Drawing for the job (mm, zero at the part's lowest x, y, z). A direction names the side the tool comes from. Coordinates: 2 decimals unless noted, no trailing zeros. Loops run counter-clockwise (first coordinate to the right, second up) from the corner with the lowest first, then second, coordinate; pieces in that order, holes last. Notation, with made-up numbers: (20.5, 40) - (59.5, 40) arc R18 cw to (59.5, 71) - close; hole circle Ø6 at (-13, -13.5). An arc over 180 degrees is marked (long way). Put each result on its own line as item: value.
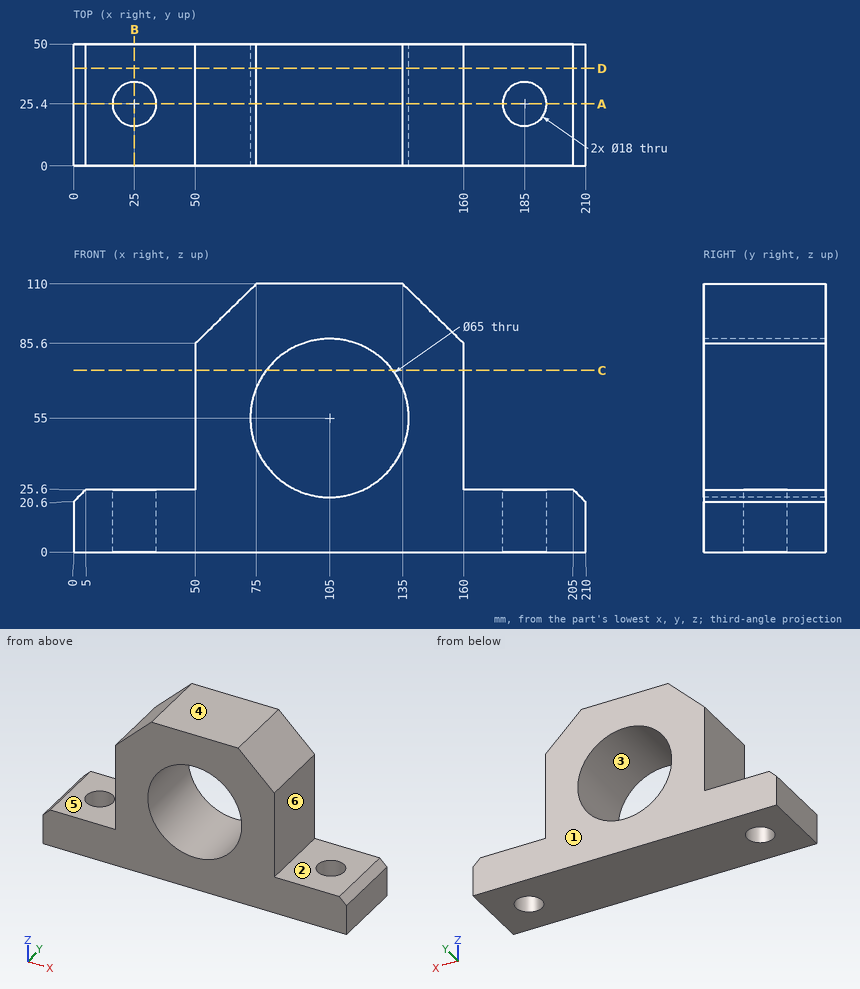
Q1. Tool access for the marked faces 4, 5 and 6: list every direction of +Z, -Z, +X, -X, +Y, -Y with a clear straight run to the whole face (end or side of a thin tool).
Determined:
face 4: +Z, +X, -X, +Y, -Y
face 5: +Z, -X, +Y, -Y
face 6: +Z, +X, +Y, -Y
Q2. Mould opens along Z. For the marked faces 1, 2 and 3 say: +Z half, -Z half, draft (parallel to the pull), parting line (faces both ways), or undercut.
Determined:
face 1: draft
face 2: +Z half
face 3: undercut
Q3. Pin check, flat tips, straight feed: pin 1 Ø13.5 at (x, y) = (21, 19.5) entering from +Z; pin 2 Ø1.5 at (y, z) = (36.5, 29) entering from -X. Stop position of each tip, or through.
Determined:
pin 1: z = 25.6
pin 2: x = 50
Q4. Slice it at C-C, the plane z = 74.5. Give the cut face in (x, y), then the cut area to 3 significant figures.
Determined:
outline: (50, 0) - (79, 0) - (79, 50) - (50, 50) - close; (131, 0) - (160, 0) - (160, 50) - (131, 50) - close
area: 2,900 mm2
Q5. Wall check: L1, parallel to Z at x = 105, y = 23.5; L2, parallel to Y at x = 185, z = 10.75; L3, parallel to Z at x = 18, y = 19. Give the ranges that are in metal, low to high. Write a range as from..to.
Determined:
L1: 0..22.5, 87.5..110
L2: 0..16.4, 34.4..50
L3: 0..25.6
Q6. Slice it at B-B, the plane x = 25. Give the cut face in (y, z).
Determined:
outline: (0, 0) - (16.4, 0) - (16.4, 25.6) - (0, 25.6) - close; (34.4, 0) - (50, 0) - (50, 25.6) - (34.4, 25.6) - close
Q7. Slice it at A-A, the plane y = 25.4. Give the cut face in (x, z), then the cut area to 3 significant figures.
Determined:
outline: (0, 0) - (16, 0) - (16, 25.6) - (5, 25.6) - (0, 20.6) - close; (34, 0) - (176, 0) - (176, 25.6) - (160, 25.6) - (160, 85.6) - (135, 110) - (75, 110) - (50, 85.6) - (50, 25.6) - (34, 25.6) - close; (194, 0) - (210, 0) - (210, 20.6) - (205, 25.6) - (194, 25.6) - close; hole circle Ø65 at (105, 55)
area: 9,790 mm2
Q8. Slice it at D-D, the plane y = 40. Give the cut face in (x, z).
Determined:
outline: (0, 0) - (210, 0) - (210, 20.6) - (205, 25.6) - (160, 25.6) - (160, 85.6) - (135, 110) - (75, 110) - (50, 85.6) - (50, 25.6) - (5, 25.6) - (0, 20.6) - close; hole circle Ø65 at (105, 55)
